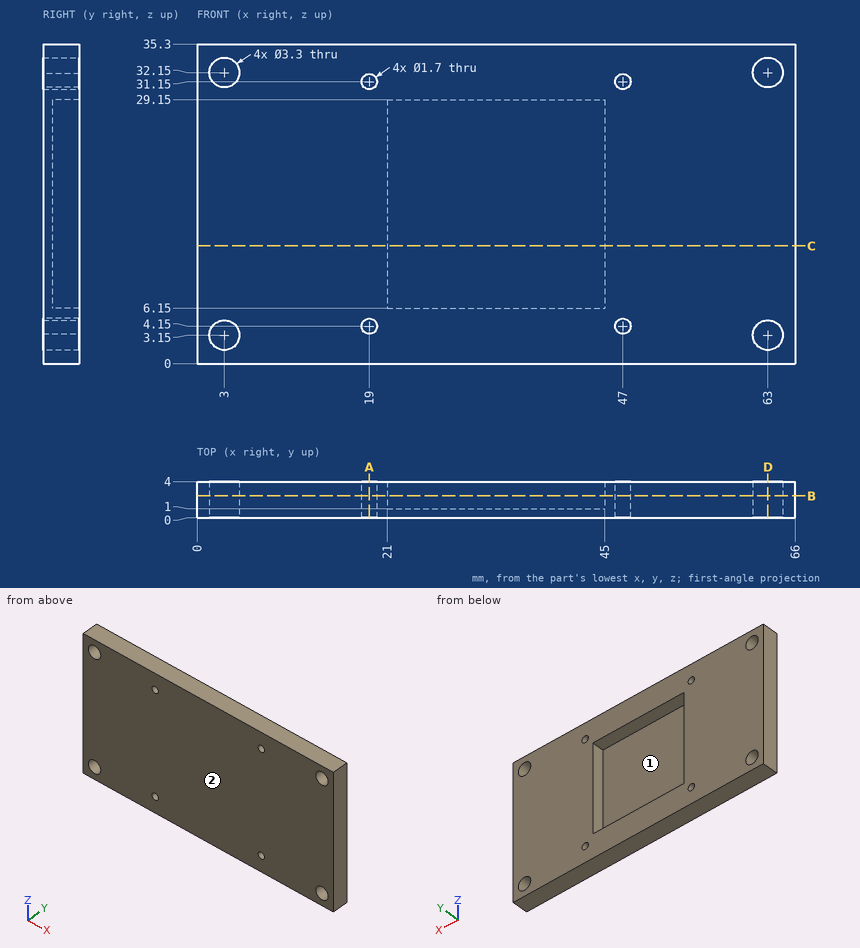
Could you check a few things on this drawing? It's one solid part, dimensions in mm from its lowest x, y, z. Round coordinates to 2 decimals unless told otherwise and drop trailing zeros. Order: outer loops, then holes, each group sorted by start corner. A loop starts at its lowest first (then second) coordinate and runs counter-clockwise, first axis right, second up. Notation, with made-up numbers: M 19,41.5 L 63,41.5 A11 cw 63,51.5 Z; hole C -20.75,40 d3. An arc over 180 degrees is marked long. One line per item, written item: value.
(1) Imagine slicing it at D-D (x = 63). Write out the boundary of the cut face in (y, z).
Ans:
outline: M 0,0 L 4,0 L 4,1.5 L 0,1.5 Z; M 0,4.8 L 4,4.8 L 4,30.5 L 0,30.5 Z; M 0,33.8 L 4,33.8 L 4,35.3 L 0,35.3 Z
(2) Imagine slicing it at A-A (x = 19). Write out the boundary of the cut face in (y, z), and give its area (3 significant figures).
Ans:
outline: M 0,0 L 4,0 L 4,3.3 L 0,3.3 Z; M 0,5 L 4,5 L 4,30.3 L 0,30.3 Z; M 0,32 L 4,32 L 4,35.3 L 0,35.3 Z
area: 128 mm^2
(3) If we mould it in two halves opening along Z, with no side actions, what happens to the marked faces 1 and 2? For each: released by +Z, released by -Z, zero draft, split by the parting line, or undercut.
Ans:
face 1: undercut
face 2: zero draft
(4) Imagine slicing it at B-B (y = 2.45). Count the separate pieces of the cut face and the enclosed holes in it, and give its area (3 significant figures).
Ans:
separate pieces: 1
enclosed holes: 9
area: 1,730 mm^2
(5) Imagine slicing it at C-C (z = 13). Write out the boundary of the cut face in (x, y).
Ans:
outline: M 0,0 L 66,0 L 66,4 L 45,4 L 45,1 L 21,1 L 21,4 L 0,4 Z
(6) I need wall thicknesses on line 1 along Z through (x, y) = (47, 0.85); line 2 along Z through (x, y) = (25, 2.7); line 3 along X through (y, z) = (1.75, 31). Which ranges of each line are inside material? Lowest first, please. Write a range as from..to.
Ans:
line 1: z = 0..3.3, 5..30.3, 32..35.3
line 2: z = 0..6.15, 29.15..35.3
line 3: x = 0..1.82, 4.18..18.16, 19.84..46.16, 47.84..61.82, 64.18..66
(7) I'm going to push flat-ended pins straight in: P1, Ø2, axis at x = 3, z = 32.15, coming from the -Y side; P2, Ø7, axis at x = 35, z = 14.5, coming from the +Y side. Where does each tip first touch, or does it pass through?
Ans:
P1: passes through
P2: stops at y = 1
